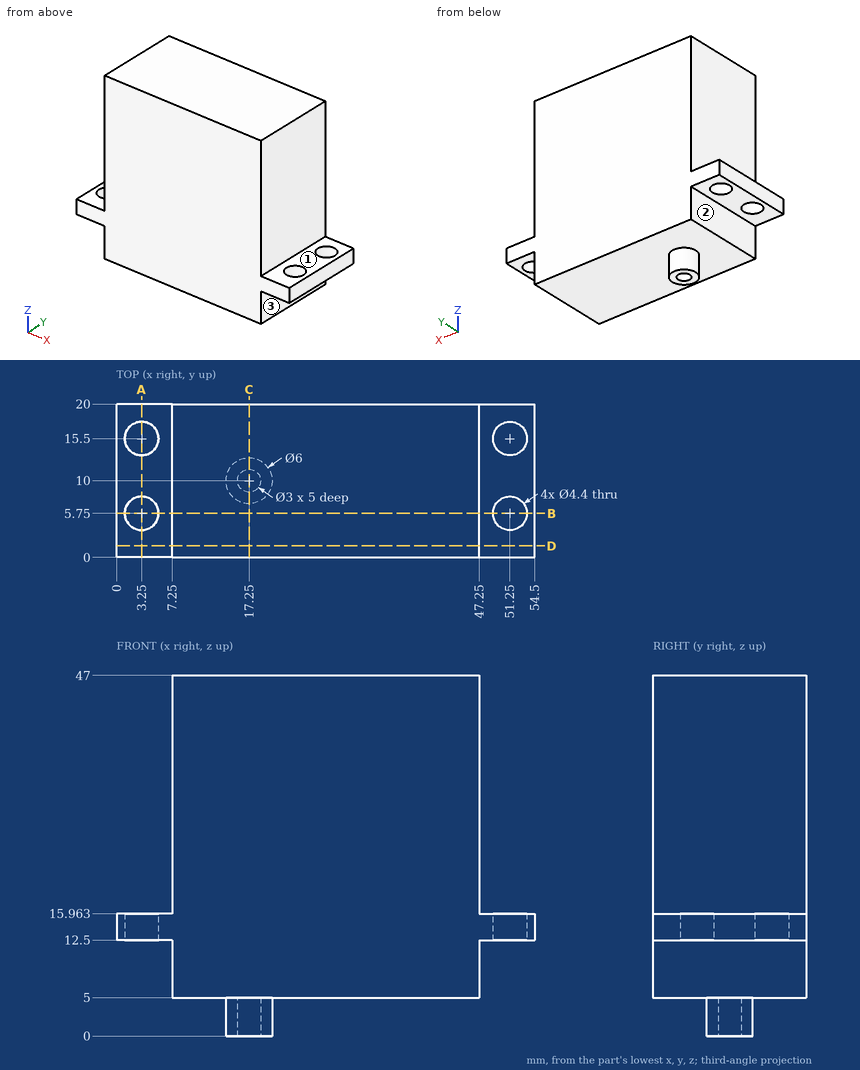
Print and shaded views of the part. All mm, measured from the part's lowest x, y and z. A direction names the side the tool comes from. Round coordinates to 2 decimals unless told otherwise and drop trailing zeros. Write each loop counter-clockwise with the first axis right and the second up, starting at its lowest first coordinate (ties: lowest second). Pieces come first, ordered by that corner, then holes. Notation, with made-up numbers: (13, 13) - (44, 13) arc R6 ccw to (44, 20) - close; hole circle Ø2 at (27, 62). An arc over 180 degrees is marked (long way). Use CSV: the item, a comma, the result in double quotes. Start each with the question number.
Item 1: Band-saw the part on B-B (y = 5.75). Write the cut outline in (x, z).
Item 2: Pin check, flat tips, straight feed: P1, Ø3, axis at x = 12.5, y = 7.5, coming from the -Z side; P2, Ø2, axis at x = 2, y = 10.5, coming from the -Z side; P3, Ø8, axis at x = 49, y = 13, coming from the +Z side; P4, Ø4, axis at y = 2.5, z = 29.5, coming from the -X side. Stop position of each tip, or through.
Item 3: Drill centre lines: L1, parallel to Y at x = 3, z = 13; L2, parallel to Z at x = 30.5, y = 18; L3, parallel to Z at x = 2, y = 18. Where is each one in solid material? Low to high. Write a range as [from, to].
Item 4: Band-saw the part on D-D (y = 1.5). Write the cut outline in (x, z), and give its area (3 significant figures).
Item 5: Band-saw the part on C-C (x = 17.25). Write the cut outline in (y, z).
Item 6: Tool access for the marked faces 1, 2 and 3: list every direction of +Z, -Z, +X, -X, +Y, -Y with a clear straight run to the whole face (end or side of a thin tool).
Item 7: Band-saw the part on A-A (x = 3.25). Write the cut outline in (y, z), and give its area (3 significant figures).
Checked values:
1,outline,"(0, 12.5) - (1.05, 12.5) - (1.05, 15.96) - (0, 15.96) - close; (5.45, 12.5) - (7.25, 12.5) - (7.25, 5) - (47.25, 5) - (47.25, 12.5) - (49.05, 12.5) - (49.05, 15.96) - (47.25, 15.96) - (47.25, 47) - (7.25, 47) - (7.25, 15.96) - (5.45, 15.96) - close; (53.45, 12.5) - (54.5, 12.5) - (54.5, 15.96) - (53.45, 15.96) - close"
2,P1,"stops at z = 5"
2,P2,"stops at z = 12.5"
2,P3,"stops at z = 47"
2,P4,"stops at x = 7.25"
3,L1,"y = [0, 3.56], [7.94, 13.31], [17.69, 20]"
3,L2,"z = [5, 47]"
3,L3,"z = [12.5, 15.96]"
4,outline,"(0, 12.5) - (7.25, 12.5) - (7.25, 5) - (47.25, 5) - (47.25, 12.5) - (54.5, 12.5) - (54.5, 15.96) - (47.25, 15.96) - (47.25, 47) - (7.25, 47) - (7.25, 15.96) - (0, 15.96) - close"
4,area,"1,730 mm²"
5,outline,"(0, 5) - (7, 5) - (7, 0) - (8.5, 0) - (8.5, 5) - (11.5, 5) - (11.5, 0) - (13, 0) - (13, 5) - (20, 5) - (20, 47) - (0, 47) - close"
6,face 1,"+Z, +X, +Y, -Y"
6,face 2,"-Z, -X, +Y, -Y"
6,face 3,"-Z, +X, +Y, -Y"
7,outline,"(0, 12.5) - (3.55, 12.5) - (3.55, 15.96) - (0, 15.96) - close; (7.95, 12.5) - (13.3, 12.5) - (13.3, 15.96) - (7.95, 15.96) - close; (17.7, 12.5) - (20, 12.5) - (20, 15.96) - (17.7, 15.96) - close"
7,area,"38.8 mm²"
